Geometry check sheet. Reference: the model listing, model coordinates, mm. Face numbers are marked on the shaded views. Round coordinates to 2 decimals unless told otherwise and drop trailing zeros. Order: outer loops, then holes, each group sorted by start corner. A loop starts at its lowest first (then second) coordinate and runs counter-clockwise, first axis right, second up. Notation, with made-up numbers: (53, 64.5) - (60, 64.5) arc R19 ccw to (60, 100.5) - close; hole circle Ø6 at (48.5, 27.25). An arc over 180 degrees is marked (long way). Write each question's results on one line, items separated by ' | '.
```python
from build123d import *

# Parameters (mm, degrees)
BOSS_EXTRUDE1_START = 12.7
SKETCH3_R           = 19.05
SKETCH3_R_2         = 12.7
BOSS_EXTRUDE1_DEPTH = 3.175
BOSS_EXTRUDE2_START = 9.525
SKETCH4_R           = 15.8877
SKETCH4_R_2         = 12.7
BOSS_EXTRUDE2_DEPTH = 22.225
CHAMFER1_SIZE       = 0.381


with BuildPart() as part:
    # Sketch3 → Boss-Extrude1 (new body)
    with BuildSketch(Plane.XY.offset(BOSS_EXTRUDE1_START)):
        Circle(SKETCH3_R)
        Circle(SKETCH3_R_2, mode=Mode.SUBTRACT)
    extrude(amount=-BOSS_EXTRUDE1_DEPTH)

    # Sketch4 → Boss-Extrude2 (add)
    with BuildSketch(Plane.XY.offset(BOSS_EXTRUDE2_START)):
        Circle(SKETCH4_R)
        Circle(SKETCH4_R_2, mode=Mode.SUBTRACT)
    extrude(amount=-BOSS_EXTRUDE2_DEPTH)

    # Chamfer1
    chamfer1_edges = [part.edges().sort_by_distance(p)[0] for p in [
        (-12.7, 0, -12.7),
        (-15.8877, 0, 9.525),
        (-19.05, 0, 12.7),
        (-19.05, 0, 9.525),
        (-12.7, 0, 12.7),
        (-15.8877, 0, -12.7),
    ]]
    chamfer(chamfer1_edges, length=CHAMFER1_SIZE)


solid = part.part
```
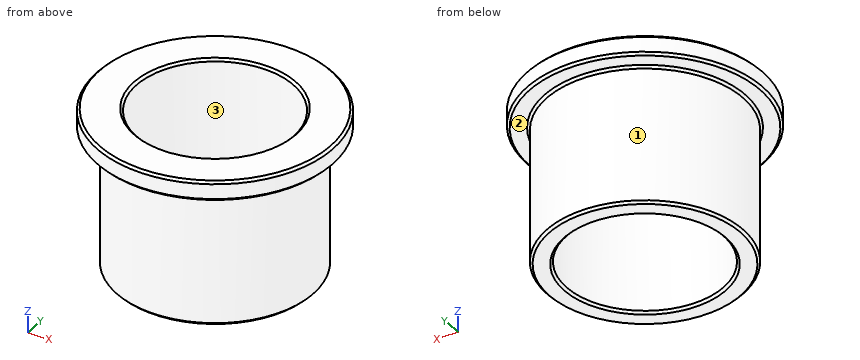
(1) Section check C-C (z = 6.75). Record the cut outline in (x, y).
Answers follow:
outline: circle Ø31.78 at (0, 0); hole circle Ø25.4 at (0, 0)
(2) Material ranges on line 1 (Y direction, x = 0, z = 0.5); line 2 (X direction, y = 6, z = -3); line 3 (X direction, y = 0.5, z = 8.25), recorded low to high.
Answers follow:
line 1: -15.89 to -12.7, 12.7 to 15.89 | line 2: -14.71 to -11.19, 11.19 to 14.71 | line 3: -15.88 to -12.69, 12.69 to 15.88
(3) Section check A-A (x = 0). Record the cut outline in (y, z) (3 decimals), then the cut area to 3 significant figures.
Answers follow:
outline: (-19.05, 9.906) - (-18.669, 9.525) - (-16.269, 9.525) - (-15.888, 9.144) - (-15.888, -12.319) - (-15.507, -12.7) - (-13.081, -12.7) - (-12.7, -12.319) - (-12.7, 12.319) - (-13.081, 12.7) - (-18.669, 12.7) - (-19.05, 12.319) - close; (12.7, -12.319) - (13.081, -12.7) - (15.507, -12.7) - (15.888, -12.319) - (15.888, 9.144) - (16.269, 9.525) - (18.669, 9.525) - (19.05, 9.906) - (19.05, 12.319) - (18.669, 12.7) - (13.081, 12.7) - (12.7, 12.319) - close | area: 181 mm²
(4) Draft check along Y on the marked faces 1, 2 and 3. Enter one of: released by +Y, released by -Y, zero draft, split by the parting line, or undercut.
Answers follow:
face 1: split by the parting line | face 2: zero draft | face 3: undercut
(5) Depth check by flat-ended pin: pin 1 Ø6 at (x, z) = (-11.5, -9) entering from +Y; pin 2 Ø6 at (x, z) = (-10.5, -6) entering from +Y; pin 3 Ø3 at (y, z) = (4.5, -1.5) entering from -X. Enter the tip coordinate at first touch or a pass-through.
Answers follow:
pin 1: y = 13.42 | pin 2: y = 14.01 | pin 3: x = -15.6
